Here's the drawing with two shaded views (mm, measured from the low corner). I have some questions. Give positions to 0.01 mm unless a question says otherwise; leave off trailing zeros. Loops run counter-clockwise (first coordinate to the right, second up) from the corner with the lowest first, then second, coordinate; pieces in that order, holes last. Notation, with made-up numbers: (46, 65.5) -> (63, 65.5) arc R9 ccw to (63, 82.5) -> close; hole circle Ø2 at (-24, 69). An arc over 180 degrees is marked (long way). Answer in a Markdown table with one row per item. Add a question column.
Item 1: For P1, Ø2, axis at y = 5, z = 34, coming from the +X side; P2, Ø8, axis at x = 12, z = 80, coming from the -Y side; P3, Ø5, axis at x = 14.5, z = 34.5, coming from the +Y side, each with a flat end and sliding along its axis, tell me the tip position at first contact or that it passes through.
Item 2: If I drill on line 1 (Z direction, x = 2, y = 6.25); line 2 (Z direction, x = 5.75, y = 11.5); line 3 (Y direction, x = 5.75, z = 33), over which ranges is the centre line in solid material (lowest first)?
Item 3: If we section it at C-C (z = 63): Write out the boundary of the cut face in (x, y), then the cut area to 3 significant figures.
Item 4: If we section it at A-A (y = 8.5): Write out the boundary of the cut face in (x, z).
Item 5: If we section it at B-B (x = 8.5): Write out the boundary of the cut face in (y, z).
Item 6: We'd pull the mould along Y, two halves only. Please class the marked faces 1 and 2: released by +Y, released by -Y, zero draft, split by the parting line, or undercut.
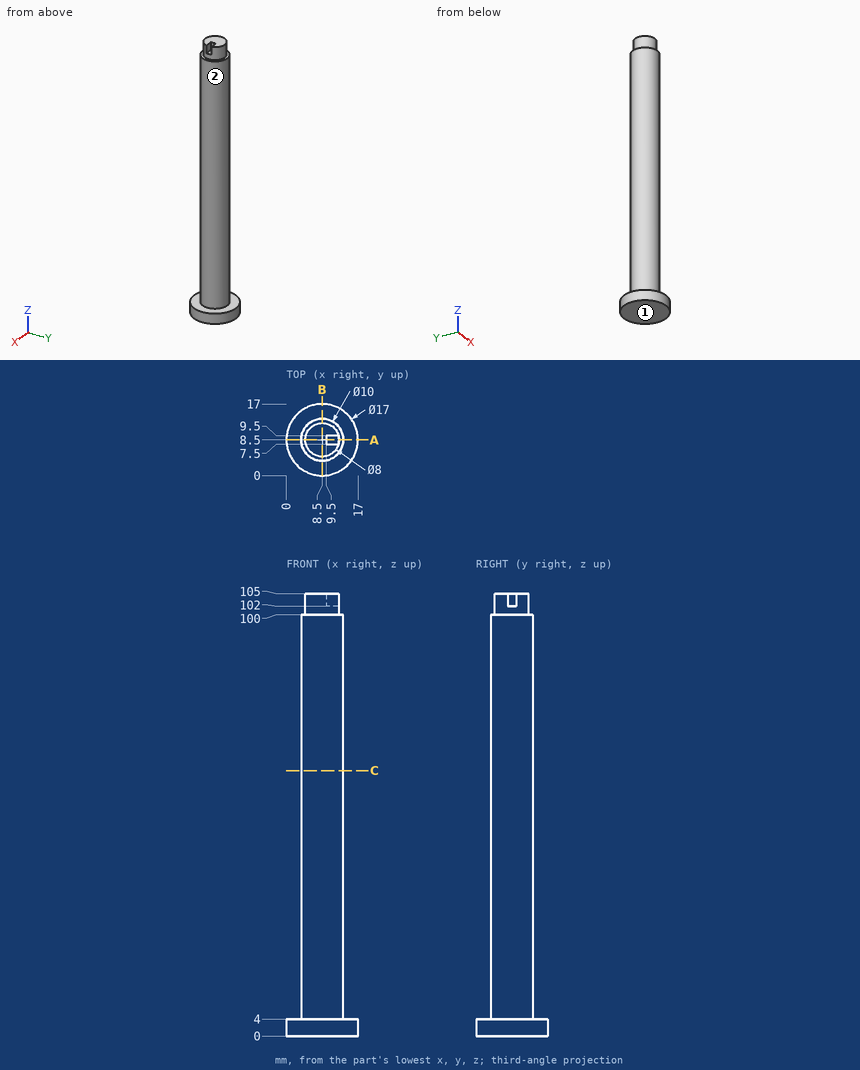
Recorded:
| question | item | result |
|---|---|---|
| 1 | P1 | stops at x = 12.83 |
| 1 | P2 | stops at y = 3.5 |
| 1 | P3 | stops at y = 12.07 |
| 2 | line 1 | z = 0 to 4 |
| 2 | line 2 | z = 0 to 100 |
| 2 | line 3 | y = 4.32 to 12.68 |
| 3 | outline | circle Ø10 at (8.5, 8.5) |
| 3 | area | 78.5 mm^2 |
| 4 | outline | (0, 0) -> (17, 0) -> (17, 4) -> (13.5, 4) -> (13.5, 100) -> (12.5, 100) -> (12.5, 102) -> (9.5, 102) -> (9.5, 105) -> (4.5, 105) -> (4.5, 100) -> (3.5, 100) -> (3.5, 4) -> (0, 4) -> close |
| 5 | outline | (0, 0) -> (17, 0) -> (17, 4) -> (13.5, 4) -> (13.5, 100) -> (12.5, 100) -> (12.5, 105) -> (4.5, 105) -> (4.5, 100) -> (3.5, 100) -> (3.5, 4) -> (0, 4) -> close |
| 6 | face 1 | zero draft |
| 6 | face 2 | split by the parting line |
